Geometry: final body of the model. Coordinates: model frame, mm. A direction names the side the tool comes from. Give positions to 0.01 mm unless a question says otherwise; leave off trailing zeros. Loops run counter-clockwise (first coordinate to the right, second up) from the corner with the lowest first, then second, coordinate; pieces in that order, holes last.
1. Material intervals for line 1 along Y through (x, z) = (-434, -17) (3 decimals); line 2 along Z through (x, y) = (-202.5, 29) (3 decimals), sorted ascending.
2. First-contact query: P1, Ø5, axis at x = -133.5, y = 31.5, coming from the -Z side (3 decimals). Flat tip, straight axial feed; report the tip coordinate or a pass-through.
3. Access query for faces 1 (the face through (-263, 0, -9)), 2 (the face through (-263, 34.925, -14)). Directions: +Z, -Z, +X, -X, +Y, -Y. A direction counts if a zero-diameter tool reaches every point of the face in a straight line with its end or side. Return the directions, or none.
4. Section A-A, the plane z = -14.25. Output: boundary loops of the cut face in (x, y) (3 decimals), then the cut area to 3 significant figures.
5. Section B-B, the plane x = -286.5. Output: boundary loops of the cut face in (y, z) (3 decimals).
6. Section C-C, the plane y = 30. Output: boundary loops of the cut face in (x, z) (3 decimals), then the cut area to 3 significant figures.
Autodesk Inventor part; units mm, degrees
ref_plane "YZ Plane" through (0, 0, 0) normal (1, 0, 0) x (0, 1, 0)
ref_plane "XZ Plane" through (0, 0, 0) normal (0, 1, 0) x (-1, 0, 0)
ref_plane "XY Plane" through (0, 0, 0) normal (0, 0, 1) x (1, 0, 0)
sketch "Sketch1" plane through (0, 0, 0) normal (0, 0, 1) x (1, 0, 0)
  line L0 (0, 0) -> (-533.4, 0)
  line L1 (-533.4, 0) -> (-533.4, 47.625)
  line L2 (-533.4, 47.625) -> (0, 47.625)
  line L3 (0, 47.625) -> (0, 0)
  dimension "d0" = 533.4
  dimension "d1" = 47.625
  dimension "d2" = 0
  dimension "d3" = 0
extrude "Extrusion1" add sketch "Sketch1" against normal blind 19.05
sketch "Sketch2" plane through (0, 0, 0) normal (1, 0, 0) x (0, 0, -1)
  line L0 (0, 0) -> (19.05, 0)
  line L1 (0, 47.625) -> (19.05, 47.625)
  line L2 (19.05, 47.625) -> (19.05, 0)
  line L3 (19.05, 0) -> (0, 0)
  line L4 (0, 0) -> (0, 47.625)
  line L5 (19.05, 34.925) -> (9.525, 34.925)
  line L6 (9.525, 34.925) -> (9.525, 25.4)
  line L7 (9.525, 25.4) -> (19.05, 25.4)
  line L8 (19.05, 25.4) -> (19.05, 34.925)
  dimension "d6" = 12.7
  dimension "d7" = 9.525
  dimension "d8" = 25.4
  dimension "d11" = 9.525
extrude "Extrusion2" cut sketch "Sketch2" against normal through all contours L7 L6 L5 L2
properties part number "bottom_board_side_slat" material "Wood (Birch)"
Answers below:
1. line 1: y = 0 to 25.4, 34.925 to 47.625
1. line 2: z = -9.525 to 0
2. P1: stops at z = -9.525
3. face 1: +Z, -Z, +X, -X, -Y
3. face 2: -Z, +X, -X
4. outline: (-533.4, 0) - (0, 0) - (0, 25.4) - (-533.4, 25.4) - close; (-533.4, 34.925) - (0, 34.925) - (0, 47.625) - (-533.4, 47.625) - close
4. area: 20,300 mm2
5. outline: (0, -19.05) - (25.4, -19.05) - (25.4, -9.525) - (34.925, -9.525) - (34.925, -19.05) - (47.625, -19.05) - (47.625, 0) - (0, 0) - close
6. outline: (-533.4, -9.525) - (0, -9.525) - (0, 0) - (-533.4, 0) - close
6. area: 5,080 mm2
